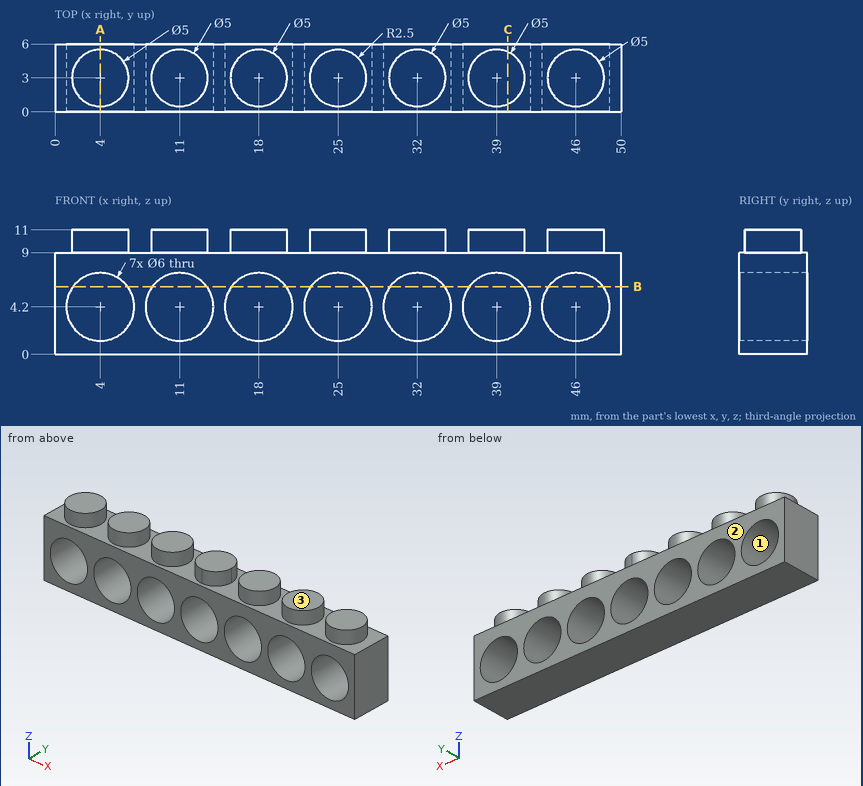
Geometry: see drawing. Coordinates: mm, zero at the bounding-box minimum. Give positions to 0.01 mm unless a question says otherwise; leave off trailing zeros. Write each loop counter-clockwise with the first axis right and the second up, starting at its lowest first coordinate (ties: lowest second). Pieces come first, ordered by that corner, then holes. Notation, with made-up numbers: (58.5, 67) - (65.5, 67) arc R22 cw to (65.5, 96) - close; hole circle Ø9 at (50.5, 34). An arc over 180 degrees is marked (long way). Return JSON: item names as keys, results as strings. Group by question number.
1) Mould query, pull axis Z, two halves, no side actions, for the marked faces 1, 2 and 3. Classes: released by +Z, released by -Z, zero draft, split by the parting line, or undercut.
2) Section C-C on x = 40. Return the cut outline in (y, z).
3) Section A-A on x = 4. Return the cut outline in (y, z), plus the area to 3 significant figures.
4) First-contact query: P1, Ø5.5, axis at x = 46, z = 4.2, coming from the -Y side; P2, Ø1.8, axis at x = 28.5, y = 1.5, coming from the +Z side. Flat tips, straight axial feed; report the tip coordinate or a pass-through.
5) Section B-B on z = 6. State how many separate pieces and enclosed holes the cut face has, plus the area to 3 significant figures.
6) Line query: line 1 (Z direction, x = 32, y = 3.65); line 2 (Z direction, x = 7.5, y = 5.15); line 3 (Z direction, x = 15.5, y = 4.9). Output: solid intervals per line, ascending.
Filled in:
{
 "1": {"face 1": "undercut", "face 2": "zero draft", "face 3": "released by +Z"},
 "2": {"outline": "(0, 0) - (6, 0) - (6, 1.37) - (0, 1.37) - close; (0, 7.03) - (6, 7.03) - (6, 9) - (5.29, 9) - (5.29, 11) - (0.71, 11) - (0.71, 9) - (0, 9) - close"},
 "3": {"outline": "(0, 0) - (6, 0) - (6, 1.2) - (0, 1.2) - close; (0, 7.2) - (6, 7.2) - (6, 9) - (5.5, 9) - (5.5, 11) - (0.5, 11) - (0.5, 9) - (0, 9) - close", "area": "28.0 mm^2"},
 "4": {"P1": "passes through", "P2": "stops at z = 9"},
 "5": {"separate pieces": "8", "enclosed holes": "0", "area": "98.4 mm^2"},
 "6": {"line 1": "z = 0 to 1.2, 7.2 to 11", "line 2": "z = 0 to 9", "line 3": "z = 0 to 2.54, 5.86 to 9"}
}
